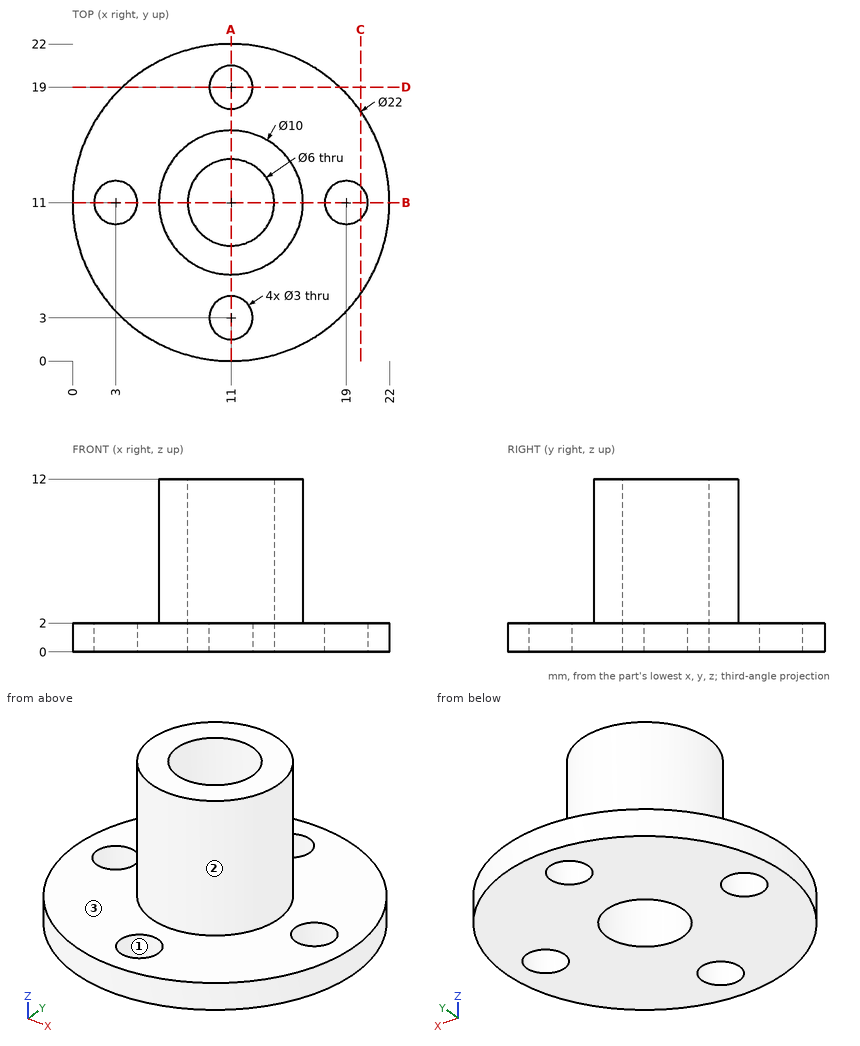
Print and shaded views of the part. All mm, measured from the part's lowest x, y and z. Round coordinates to 2 decimals unless told otherwise and drop trailing zeros. Order: outer loops, then holes, each group sorted by start corner. A loop starts at its lowest first (then second) coordinate and runs counter-clockwise, first axis right, second up.
Q1. Two-plate mould, pull along Y, no slides. Class the marked faces 1, 2 and 3: pulls with the +Y half, pulls with the -Y half, needs draft (parallel to the pull), parting line crosses it, or undercut.
Q2. Wall check: L1, parallel to Y at x = 11, z = 1.25; L2, parallel to Z at x = 17.5, y = 10.5; L3, parallel to Y at x = 11, z = 8.5. Give the ranges that are in metal, low to high.
Q3. Slice it at A-A (x = 11). Write the cut outline in (y, z), and give its area (3 significant figures).
Q4. Drop flat-ended pins along their axis: pin 1 (3 mm diameter, centred on y = 11, z = 5.5, fed in from +X); pin 2 (4 mm diameter, centred on x = 10.5, z = 8, fed in from +Y); pin 3 (2.5 mm diameter, centred on x = 3, y = 11, fed in from +Z); pin 4 (3.5 mm diameter, centred on x = 11, y = 3, fed in from +Z). Give the stop position or say it passes through.
Q5. Slice it at C-C (x = 20). Write the cut outline in (y, z), and give its area (3 significant figures).
Q6. Slice it at D-D (y = 19). Write the cut outline in (x, z).
Results below:
1. face 1: undercut
1. face 2: parting line crosses it
1. face 3: needs draft
2. L1: y = 0 to 1.5, 4.5 to 8, 14 to 17.5, 20.5 to 22
2. L2: z = 0 to 2
2. L3: y = 6 to 8, 14 to 16
3. outline: (0, 0) - (1.5, 0) - (1.5, 2) - (0, 2) - close; (4.5, 0) - (8, 0) - (8, 12) - (6, 12) - (6, 2) - (4.5, 2) - close; (14, 0) - (17.5, 0) - (17.5, 2) - (16, 2) - (16, 12) - (14, 12) - close; (20.5, 0) - (22, 0) - (22, 2) - (20.5, 2) - close
3. area: 60.0 mm2
4. pin 1: stops at x = 16
4. pin 2: stops at y = 16
4. pin 3: passes through
4. pin 4: stops at z = 2
5. outline: (4.68, 0) - (9.88, 0) - (9.88, 2) - (4.68, 2) - close; (12.12, 0) - (17.32, 0) - (17.32, 2) - (12.12, 2) - close
5. area: 20.8 mm2
6. outline: (3.45, 0) - (9.5, 0) - (9.5, 2) - (3.45, 2) - close; (12.5, 0) - (18.55, 0) - (18.55, 2) - (12.5, 2) - close
